Could you check a few things on this model? Use its own coordinates, in mm. A direction names the side the tool comes from. Give positions to 0.01 mm unless a question says otherwise; leave off trailing zeros. Write each loop counter-clockwise with the first axis right and the second up, starting at its lowest first coordinate (ties: lowest second). Pieces come first, ordered by that corner, then holes. Notation, with made-up numbers: M 36,29 L 48,29 A14 cw 48,33 Z; hole C 58.25,38 d6. An arc over 180 degrees is marked long. Use one line per item in the form item = value.
from build123d import *

# Parameters (mm, degrees)
SKETCH1_R          = 1.4224
EXTRUDE1_DEPTH     = 9.525
CHAMFER3_SIZE      = 0.47625
SKETCH6_R          = 2.3241
EXTRUDE2_DEPTH     = 2.8448
CUT_EXTRUDE1_DEPTH = 1.7859375
CHAMFER1_SIZE      = 0.23241
CHAMFER2_SIZE      = 0.116205


with BuildPart() as part:
    # Sketch1 → Extrude1 (new body)
    with BuildSketch(Plane.XY):
        Circle(SKETCH1_R)
    extrude(amount=-EXTRUDE1_DEPTH)

    # Chamfer3
    chamfer3_edges = [part.edges().sort_by_distance(p)[0] for p in [
        (-1.4224, 0, 0),
    ]]
    chamfer(chamfer3_edges, length=CHAMFER3_SIZE)

    # Sketch6 → Extrude2 (add)
    with BuildSketch(Plane(origin=(0, 0, -9.525), x_dir=(-1, 0, 0), z_dir=(0, 0, -1))):
        Circle(SKETCH6_R)
    extrude(amount=EXTRUDE2_DEPTH)

    # Sketch7 → Cut-Extrude1 (cut)
    with BuildSketch(Plane(origin=(0, 0, -12.3698), x_dir=(-1, 0, 0), z_dir=(0, 0, -1))):
        Polygon((0, 1.374815329), (-1.190625, 0.687407664), (-1.190625, -0.687407664), (0, -1.374815329), (1.190625, -0.687407664), (1.190625, 0.687407664), align=None)
    extrude(amount=-CUT_EXTRUDE1_DEPTH, mode=Mode.SUBTRACT)

    # Cut-Extrude2 cone 1 section (through the dimple's axis) → Cut-Extrude2 (revolve, cut)
    with BuildSketch(Plane(origin=(0, 0, -12.3698), x_dir=(0, 1, 0), z_dir=(1, 0, 0))):
        Polygon((0, 0), (1.374815329, 0), (0, 1.374815329), align=None)
    revolve(axis=Axis((0, 0, -12.3698), (0, 0, 1)), mode=Mode.SUBTRACT)

    # Chamfer1
    chamfer1_edges = [part.edges().sort_by_distance(p)[0] for p in [
        (2.3241, 0, -12.3698),
    ]]
    chamfer(chamfer1_edges, length=CHAMFER1_SIZE)

    # Chamfer2
    chamfer2_edges = [part.edges().sort_by_distance(p)[0] for p in [
        (2.3241, 0, -9.525),
    ]]
    chamfer(chamfer2_edges, length=CHAMFER2_SIZE)


solid = part.part
1) If I drill on L1, parallel to Z at x = -1.1, y = -1.15 (3 decimals); L2, parallel to Z at x = -0.15, y = 0.6; L3, parallel to Y at x = 0.6, z = -11, over which ranges is the centre line in solid material (lowest first)?
Checked values:
L1 = -12.37 to -9.525
L2 = -10.58 to 0
L3 = -2.25 to -1.03, 1.03 to 2.25
2) I want a section at B-B, the plane z = -2.75. Please give me the cut outline in (x, y), plus the area to 3 significant figures.
Checked values:
outline = C 0,0 d2.84
area = 6.36 mm2
3) For faces 1 (the flat face through (1.191, 0, -11)), 2 (the cylindrical face through (0.5, -2.27, -10.87)), which set-ups out of +Z, -Z, +X, -X, +Y, -Y let a thin tool reach every point of the face, with its end or its side?
Checked values:
face_1 = -Z
face_2 = +Z, -Z
4) Thinking about a two-plate mould opening in Y: for faces 3 (the flat face through (-0.6, 1.03, -11.49)), 4 (the flat face through (0, 0, 0)), 5 (the cylindrical face through (-0.31, -1.39, -4.94)), which applies, released by +Y, released by -Y, zero draft, split by the parting line, or undercut?
Checked values:
face_3 = undercut
face_4 = zero draft
face_5 = split by the parting line
5) For pin 1 Ø1.5 at (x, z) = (1.5, -4) entering from +Y; pin 2 Ø0.7 at (x, y) = (0.5, 0) entering from -Z; pin 3 Ø2 at (x, y) = (-1.5, -2) entering from +Z (3 decimals), each with a flat end and sliding along its axis, tell me the tip position at first contact or that it passes through.
Checked values:
pin_1 = 1.21
pin_2 = -10.58
pin_3 = -9.525
6) I want a section at A-A, the plane y = 0. Please give me the cut outline in (x, z) (3 decimals), plus the area to 3 significant figures.
Checked values:
outline = M -2.324,-12.137 L -2.092,-12.37 L -1.375,-12.37 L -1.191,-12.186 L -1.191,-10.584 L 1.191,-10.584 L 1.191,-12.186 L 1.375,-12.37 L 2.092,-12.37 L 2.324,-12.137 L 2.324,-9.641 L 2.208,-9.525 L 1.422,-9.525 L 1.422,-0.476 L 0.946,0 L -0.946,0 L -1.422,-0.476 L -1.422,-9.525 L -2.208,-9.525 L -2.324,-9.641 Z
area = 35.7 mm2
